Here's how the part is built. I have some questions about the finished solid (model axes, mm). A direction names the side the tool comes from. Coordinates: 2 decimals unless noted, no trailing zeros. Loops run counter-clockwise (first coordinate to the right, second up) from the corner with the lowest first, then second, coordinate; pieces in that order, holes last. Notation, with made-up numbers: (12.5, 35.5) - (26.5, 35.5) arc R28 ccw to (26.5, 67.5) - close; hole circle Ø7 at (-1.5, -29). An arc over 180 degrees is marked (long way). Use a Markdown table: item, result.
```python
from build123d import *

# Parameters (mm, degrees)
SKETCH1_W           = 127
SKETCH1_H           = 53.65
BOSS_EXTRUDE1_DEPTH = 3.5
BOSS_EXTRUDE3_DEPTH = 127
SKETCH4_R           = 1.5
CUT_EXTRUDE1_DEPTH  = 3.5
SKETCH6_R           = 1.5
CUT_EXTRUDE3_DEPTH  = 3.5
FILLET1_R           = 1.5
FILLET2_R           = 1.5


with BuildPart() as part:
    # Sketch1 → Boss-Extrude1 (new body)
    with BuildSketch(Plane.XY):
        with Locations((63.5, 26.825)):
            Rectangle(SKETCH1_W, SKETCH1_H)
    extrude(amount=BOSS_EXTRUDE1_DEPTH)

    # Sketch2 → Boss-Extrude3 (add)
    with BuildSketch(Plane.ZY):
        with BuildLine():
            Line((3.5, 53.65), (3.5, 54.15))
            ThreePointArc((3.5, 54.15), (2.621320344, 56.271320344), (0.5, 57.15))
            Line((0.5, 57.15), (-82.44, 57.15))
            Line((-82.44, 57.15), (-82.44, 53.65))
            Line((-82.44, 53.65), (0, 53.65))
            Line((0, 53.65), (3.5, 53.65))
        make_face()
    extrude(amount=-BOSS_EXTRUDE3_DEPTH)

    # Sketch4 → Cut-Extrude1 (cut)
    with BuildSketch(Plane(origin=(0, 0, 0), x_dir=(-1, 0, 0), z_dir=(0, 0, -1))):
        with Locations((-121, 39.15)):
            Circle(SKETCH4_R)
        with Locations((-121, 12.5)):
            Circle(SKETCH4_R)
        with Locations(Location((-6, 12.5, 0), (0, 0, 180))):
            Circle(SKETCH4_R)
        with Locations(Location((-6, 39.15, 0), (0, 0, 180))):
            Circle(SKETCH4_R)
    extrude(amount=-CUT_EXTRUDE1_DEPTH, mode=Mode.SUBTRACT)

    # Sketch6 → Cut-Extrude3 (cut)
    with BuildSketch(Plane.XZ.offset(-53.65)):
        with Locations(Location((6, -20.5, 0), (0, 0, 270))):
            Circle(SKETCH6_R)
        with Locations(Location((6, -64.94, 0), (0, 0, 270))):
            Circle(SKETCH6_R)
        with Locations(Location((121, -64.94, 0), (0, 0, 90))):
            Circle(SKETCH6_R)
        with Locations(Location((121, -20.5, 0), (0, 0, 90))):
            Circle(SKETCH6_R)
    extrude(amount=-CUT_EXTRUDE3_DEPTH, mode=Mode.SUBTRACT)

    # Fillet1
    fillet1_edges = [part.edges().sort_by_distance(p)[0] for p in [
        (127, 27.075, 3.5),
        (127, 57.15, -40.97),
        (127, 56.271320344, 2.621320344),
    ]]
    fillet(fillet1_edges, radius=FILLET1_R)

    # Fillet2
    fillet2_edges = [part.edges().sort_by_distance(p)[0] for p in [
        (0, 56.271320344, 2.621320344),
        (0, 57.15, -40.97),
        (0, 27.075, 3.5),
    ]]
    fillet(fillet2_edges, radius=FILLET2_R)


solid = part.part
```
Q1. I want a section at B-B, the plane x = 6. Write out the boundary of the cut face in (y, z).
Check values:
| item | result |
|---|---|
| outline | (0, 0) - (11, 0) - (11, 3.5) - (0, 3.5) - close; (14, 0) - (37.65, 0) - (37.65, 3.5) - (14, 3.5) - close; (40.65, 0) - (53.65, 0) - (53.65, -19) - (57.15, -19) - (57.15, 0.5) arc R3 ccw to (54.15, 3.5) - (40.65, 3.5) - close; (53.65, -82.44) - (57.15, -82.44) - (57.15, -66.44) - (53.65, -66.44) - close; (53.65, -63.44) - (57.15, -63.44) - (57.15, -22) - (53.65, -22) - close |
Q2. Please list where these lines run through material, in increasing order: L1, parallel to X at y = 55.95, z = -64.94; L2, parallel to Z at x = 121, y = 54; L3, parallel to Y at x = 121, z = 2.2. Write a range as from..to.
Check values:
| item | result |
|---|---|
| L1 | 0.03..4.5, 7.5..119.5, 122.5..126.97 |
| L2 | -82.44..-66.44, -63.44..-22, -19..3.5 |
| L3 | 0..11, 14..37.65, 40.65..56.62 |
Q3. Which directions (+Z, -Z, +X, -X, +Y, -Y) give clear straight access to the entire face, cutting with the end or side of a thin tool? Please do faces 5 (the face through (63, 53.65, -42)), 6 (the face through (63, 57.15, -40)).
Check values:
| item | result |
|---|---|
| face 5 | -Z, +X, -X, -Y |
| face 6 | +Z, -Z, +X, -X, +Y |
Q4. I want a section at A-A, the plane y = 12.5. Write out the boundary of the cut face in (x, z), then the cut area to 3 significant figures.
Check values:
| item | result |
|---|---|
| outline | (0, 0) - (4.5, 0) - (4.5, 3.5) - (1.5, 3.5) arc R1.5 ccw to (0, 2) - close; (7.5, 0) - (119.5, 0) - (119.5, 3.5) - (7.5, 3.5) - close; (122.5, 0) - (127, 0) - (127, 2) arc R1.5 ccw to (125.5, 3.5) - (122.5, 3.5) - close |
| area | 423 mm^2 |
Q5. If we mould it in two halves opening along X, with no side actions, what happens to faces 1 (the face through (63, 0, 2)), 2 (the face through (0, 55, -22)), 3 (the face through (122.5, 39.2, 1.7)), 4 (the face through (4.5, 12.43, 1.73))? For each: pulls with the +X half, pulls with the -X half, needs draft (parallel to the pull), parting line crosses it, or undercut.
Check values:
| item | result |
|---|---|
| face 1 | needs draft |
| face 2 | pulls with the -X half |
| face 3 | undercut |
| face 4 | undercut |
Q6. Will these pins go through, and if not, where does the flat tip stop? P1, Ø24.5, axis at x = 55, z = -51.5, coming from the -Y side; P2, Ø1.8, axis at x = 121, z = -64.94, coming from the +Y side; P3, Ø4, axis at x = 6, y = 12.5, coming from the -Z side; P4, Ø4, axis at x = 6, z = -20.5, coming from the +Y side.
Check values:
| item | result |
|---|---|
| P1 | y = 53.65 |
| P2 | through |
| P3 | z = 0 |
| P4 | y = 57.15 |
Q7. I want a section at C-C, the plane z = -64.94. Write out the boundary of the cut face in (x, y).
Check values:
| item | result |
|---|---|
| outline | (0, 53.65) - (4.5, 53.65) - (4.5, 57.15) - (1.5, 57.15) arc R1.5 ccw to (0, 55.65) - close; (7.5, 53.65) - (119.5, 53.65) - (119.5, 57.15) - (7.5, 57.15) - close; (122.5, 53.65) - (127, 53.65) - (127, 55.65) arc R1.5 ccw to (125.5, 57.15) - (122.5, 57.15) - close |
Q8. I want a section at D-D, the plane x = 114.5. Write out the boundary of the cut face in (y, z), then the cut area to 3 significant figures.
Check values:
| item | result |
|---|---|
| outline | (0, 0) - (53.65, 0) - (53.65, -82.44) - (57.15, -82.44) - (57.15, 0.5) arc R3 ccw to (54.15, 3.5) - (0, 3.5) - close |
| area | 487 mm^2 |
